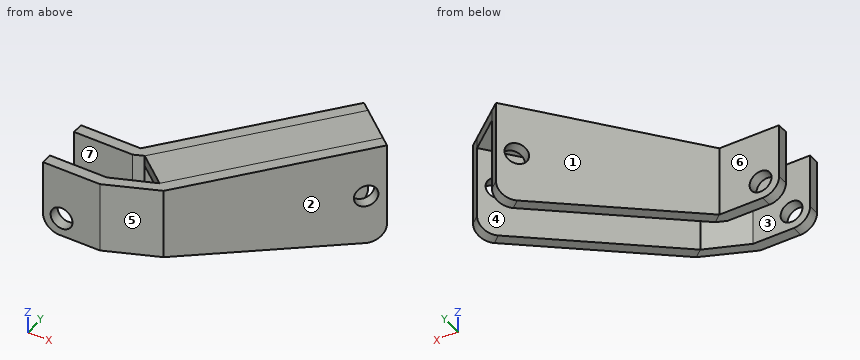
Autodesk Inventor part; units mm, degrees
ref_plane "YZ Plane" through (0, 0, 0) normal (1, 0, 0) x (0, 1, 0)
ref_plane "XZ Plane" through (0, 0, 0) normal (0, 1, 0) x (-1, 0, 0)
ref_plane "XY Plane" through (0, 0, 0) normal (0, 0, 1) x (1, 0, 0)
sketch "Esquisse1" plane through (0, 0, 0) normal (0, 0, 1) x (1, 0, 0)
  line L0 (0, 0) -> (0, 2)
  line L1 (0, 2) -> (10.4, 2)
  line L2 (0, 0) -> (10.4, 0)
  line L3 (10.4, 0) -> (19.648, 3.8307)
  line L4 (0, 9) -> (10.7082, 9)
  line L5 (0, 11) -> (0, 9)
  line L6 (0, 11) -> (10.9257, 11)
  line L7 (10.4, 2) -> (18.103, 5.1006)
  line L8 (18.103, 5.1006) -> (19.648, 3.8307)
  line L9 (10.9257, 11) -> (19.648, 3.8307) construction
  line L10 (10.9257, 11) -> (12.2416, 9.9184) construction
  line L11 (10.9257, 11) -> (12.4707, 9.73)
  line L12 (10.7082, 9) -> (12.4707, 9.73)
  dimension "d0" = 2
  dimension "d1" = 10.4
  dimension "d2" = 10.4
  dimension "d3" = 157.5
  dimension "d5" = 10.01
  dimension "d8" = 7
  dimension "d26" = 2
  dimension "d32" = 2
  dimension "d33" = 2
  dimension "d34" = 157.5
extrude "Extrusion1" add sketch "Esquisse1" along normal blind 13
sketch "Esquisse4" plane through (0, 0, 0) normal (0, -1, 0) x (1, 0, 0)
  circle A0 centre (3.39, 3.39) radius 2
  line L0 (0, 13) -> (10.4, 13)
  line L1 (0, 0) -> (0, 13)
  line L2 (10.4, 0) -> (0, 0)
  point P0 (3, 13)
  point P1 (0, 10)
  dimension "d35" = 4
  dimension "d37" = 3.39
  dimension "d50" = 3.39
extrude "Extrusion3" cut sketch "Esquisse4" against normal blind 13
ref_plane "Plan de construction3" through (19.648, 3.8307, 13) normal (-0.7725294, 0.634979, 0) x (-0.634979, -0.7725294, 0)
sketch "Esquisse5" plane through (19.648, 3.8307, 13) normal (-0.7725294, 0.634979, 0) x (-0.634979, -0.7725294, 0)
  line L0 (0, 0) -> (6.9376, 0)
  line L1 (0, -13) -> (6.9376, -13)
  line L2 (0, 0) -> (0, -13)
  line L3 (0, -13) -> (-32.924, -18.2914)
  line L4 (-36.4, -15.3294) -> (-36.4, 0)
  line L5 (-36.4, 0) -> (0, 0)
  arc A0 (-36.4, -15.3294) -> (-32.924, -18.2914) centre (-33.4, -15.3294) ccw
  point P0 (15.4354, -13)
  point P1 (5.0326, 0)
  point P2 (-36.4, -18.85)
  dimension "d40" = 36.4
  dimension "d41" = 18.85
  dimension "d42" = 3
extrude "Extrusion4" add sketch "Esquisse5" along normal blind 2
ref_plane "Plan de construction4" through (12.4707, 9.73, 13) normal (-0.7725294, 0.634979, 0) x (-0.634979, -0.7725294, 0)
sketch "Esquisse6" plane through (12.4707, 9.73, 13) normal (-0.7725294, 0.634979, 0) x (-0.634979, -0.7725294, 0)
  line L0 (0, -13) -> (0, 0)
  line L1 (0, -13) -> (0, 0)
  line L2 (0, -13) -> (0, 0)
  line L3 (0, 0) -> (-36.4, 0)
  line L4 (-36.4, 0) -> (-36.4, -15.3294)
  line L5 (-36.4, 0) -> (-36.4, -15.3294)
  line L6 (-32.924, -18.2914) -> (0, -13)
  arc A0 (-36.4, -15.3294) -> (-32.924, -18.2914) centre (-33.4, -15.3294) ccw
  point P0 (15.4354, -13)
  point P1 (-36.4, -18.85)
  dimension "d45" = 36.4
  dimension "d46" = 18.85
  dimension "d47" = 3
extrude "Extrusion5" add sketch "Esquisse6" along normal blind 2
fillet "Congé4" radius 3 2 edges at (0, 1, 0) (0, 10, 0)
ref_plane "Plan de construction6" through (34.8114, 38.4851, 13) normal (0, 0, -1) x (-1, 0, 0)
sketch "Esquisse8" plane through (34.8114, 38.4851, 13) normal (0, 0, -1) x (-1, 0, 0)
  line L0 (1.4347, -3.3203) -> (-0.7725, -0.635)
  line L1 (24.1032, -29.4851) -> (22.3407, -28.755)
  line L2 (-0.7725, -0.635) -> (22.3407, -28.755)
  line L3 (16.7085, -33.3845) -> (-6.4048, -5.2644)
  line L4 (22.3407, -28.755) -> (16.7085, -33.3845)
  line L5 (16.7085, -33.3845) -> (-6.4048, -5.2644)
  line L6 (-6.4048, -5.2644) -> (-0.7725, -0.635)
  point P0 (34.8114, -38.4851)
extrude "Extrusion6" add sketch "Esquisse8" along normal blind 2
sketch "Esquisse9" plane through (19.648, 3.8307, 13) normal (0.7725294, -0.634979, 0) x (0, 0, -1)
  circle A0 centre (9.1, 33.01) radius 2
  line L0 (18.2914, 32.924) -> (13, 0) construction
  line L1 (17.0751, 25.3561) -> (18.85, 36.4) construction
  line L2 (18.85, 36.4) -> (0, 36.4) construction
  line L3 (0, 36.4) -> (0, 0) construction
  point P0 (13, -15.4354)
  dimension "d54" = 3.39
  dimension "d55" = 9.1
  dimension "d56" = 4
extrude "Extrusion7" cut sketch "Esquisse9" against normal blind 13
properties part number "Thumb1" material "Plastique ABS"
Part model, mm, in its own coordinate system. Face numbers are marked on the shaded views. A direction names the side the tool comes from. Round coordinates to 2 decimals unless told otherwise and drop trailing zeros. Loops run counter-clockwise (first coordinate to the right, second up) from the corner with the lowest first, then second, coordinate; pieces in that order, holes last. Notation, with made-up numbers: (-18.75, 71) -> (-3.75, 71) arc R26 ccw to (-3.75, 85) -> close; hole circle Ø2 at (49.5, 48.25). An arc over 180 degrees is marked (long way). Use one line per item in the form item = value. Start each with the question number.
Item 1: Tool access for the marked faces 5, 6 and 7: list every direction of +Z, -Z, +X, -X, +Y, -Y with a clear straight run to the whole face (end or side of a thin tool).
Item 2: Two-plate mould, pull along Y, no slides. Class the marked faces 1, 2, 3 and 4: released by +Y, released by -Y, zero draft, split by the parting line, or undercut.
Item 3: Band-saw the part on D-D (x = 25). List the corners of the cut face in (y, z), plus the area to 3 significant figures.
Item 4: Drop flat-ended pins along their axis: pin 1 Ø1 at (x, z) = (19.5, -3.5) entering from -Y; pin 2 Ø5 at (y, z) = (29.5, -3) entering from +X; pin 3 Ø5.5 at (x, z) = (5.5, 5.5) entering from +Y; pin 4 Ø0.6 at (x, y) = (8, 10) entering from -Z. Give the stop position or say it passes through.
Item 5: Band-saw the part on C-C (y = 17). List the corners of the cut face in (x, z).
Item 6: Drill centre lines: line 1 along Z through (x, y) = (3.39, 10.55); line 2 along Y through (x, z) = (10, 2.25); line 3 along Z through (x, y) = (32, 27.5). Where is each one in solid material? Low to high.
Item 7: Band-saw the part on A-A (z = 7). List the corners of the cut face in (x, y).
Item 8: Band-saw the part on B-B (x = 8). List the corners of the cut face in (y, z).
Data:
q1.face_5 = +Z, -Z, +X, -Y
q1.face_6 = +Z, -Z, -X, +Y
q1.face_7 = +Z, -Z, -X
q2.face_1 = released by +Y
q2.face_2 = released by -Y
q2.face_3 = undercut
q2.face_4 = undercut
q3.outline = (10.34, -1.35) -> (13.49, -1.75) -> (13.49, 11) -> (24.97, 11) -> (24.97, -3.17) -> (28.12, -3.56) -> (28.12, 13) -> (10.34, 13) -> close
q3.area = 120 mm^2
q4.pin_1 = through
q4.pin_2 = 42.76
q4.pin_3 = 11
q4.pin_4 = 0
q5.outline = (15.86, -1.25) -> (18.45, -1.51) -> (18.45, 11) -> (27.88, 11) -> (27.88, -2.48) -> (30.47, -2.74) -> (30.47, 13) -> (15.86, 13) -> close
q6.line_1 = 0 to 1.39, 5.39 to 13
q6.line_2 = 0 to 2, 9 to 11
q6.line_3 = 11 to 13
q7.outline = (0, 0) -> (10.4, 0) -> (19.65, 3.83) -> (42.76, 31.95) -> (41.22, 33.22) -> (18.1, 5.1) -> (10.4, 2) -> (0, 2) -> close; (0, 9) -> (10.71, 9) -> (12.47, 9.73) -> (35.58, 37.85) -> (34.04, 39.12) -> (10.93, 11) -> (0, 11) -> close
q8.outline = (0, 0) -> (2, 0) -> (2, 13) -> (0, 13) -> close; (9, 0) -> (11, 0) -> (11, 13) -> (9, 13) -> close
